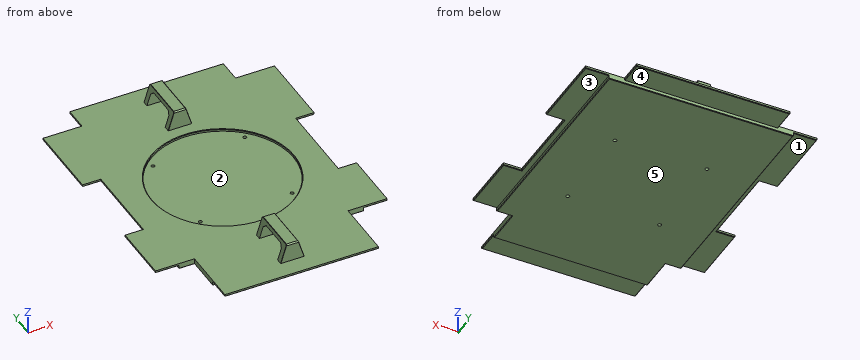
```python
from build123d import *
from OCP.BRepFilletAPI import BRepFilletAPI_MakeChamfer

# Parameters (mm, degrees)
SKETCH_1_W          = 156
SKETCH_1_H          = 185
EXTRUDE_1_DEPTH     = 3
SKETCH_2_W          = 130
SKETCH_2_H          = 30
EXTRUDE_2_DEPTH     = 3
EXTRUDE_3_DEPTH     = 2
SKETCH_4_W          = 15.5
SKETCH_4_H          = 50
SKETCH_4_H_2        = 65
EXTRUDE_4_DEPTH     = 2
SKETCH_5_R          = 1.5
CUT_EXTRUDE_1_DEPTH = 174.018062641
CHAMFER_1_SIZE      = 0.5
CHAMFER_2_SIZE      = 0.5
CHAMFER_3_SIZE      = 0.5
SKETCH_6_R          = 60
CUT_EXTRUDE_2_DEPTH = 2
CHAMFER_4_SIZE      = 0.5
EXTRUDE_5_DEPTH     = 10
CUT_EXTRUDE_3_DEPTH = 261.086524065
CHAMFER_5_SIZE      = 3
CHAMFER_6_SIZE      = 1
CHAMFER_7_SIZE      = 0.2
CHAMFER_7_SIZE2     = 0.159648139
CHAMFER_7_SIZE2_2   = 0.168291059
CHAMFER_7_SIZE2_3   = 0.304782811
CHAMFER_7_SIZE2_4   = 0.260894728


with BuildPart() as part:
    # 草图1 → 凸台-拉伸1 (new body)
    with BuildSketch(Plane.XY):
        Rectangle(SKETCH_1_W, SKETCH_1_H)
    extrude(amount=EXTRUDE_1_DEPTH)

    # 草图2 → 凸台-拉伸2 (add)
    with BuildSketch(Plane.XY.offset(3)):
        with Locations((0, -107.5)):
            Rectangle(SKETCH_2_W, SKETCH_2_H)
    extrude(amount=-EXTRUDE_2_DEPTH)

    # 草图3 → 凸台-拉伸3 (add)
    with BuildSketch(Plane.XY.offset(3)):
        Polygon((-82.5, 92.5), (-65, 92.5), (-65, 112.5), (65, 112.5), (65, 92.5), (82.5, 92.5), (82.5, -92.5), (65, -92.5), (65, -142.5), (-65, -142.5), (-65, -92.5), (-82.5, -92.5), align=None)
    extrude(amount=EXTRUDE_3_DEPTH)

    # 草图4 → 凸台-拉伸4 (add)
    with BuildSketch(Plane.XY.offset(5)):
        with Locations((-90.25, -67.5)):
            Rectangle(SKETCH_4_W, SKETCH_4_H)
        with Locations((-90.25, 60)):
            Rectangle(SKETCH_4_W, SKETCH_4_H_2)
        with Locations((90.25, 60)):
            Rectangle(SKETCH_4_W, SKETCH_4_H_2)
        with Locations((90.25, -67.5)):
            Rectangle(SKETCH_4_W, SKETCH_4_H)
    extrude(amount=-EXTRUDE_4_DEPTH)

    # 草图5 → 切除-拉伸1 (cut, through all)
    with BuildSketch(Plane.XY.offset(5)):
        with Locations((-38.890872965, 26.390872965)):
            Circle(SKETCH_5_R)
        with Locations((38.890872965, 26.390872965)):
            Circle(SKETCH_5_R)
        with Locations((38.890872965, -51.390872965)):
            Circle(SKETCH_5_R)
        with Locations((-38.890872965, -51.390872965)):
            Circle(SKETCH_5_R)
    extrude(amount=-CUT_EXTRUDE_1_DEPTH, mode=Mode.SUBTRACT)

    # 倒角1
    chamfer_1_edges = [part.edges().sort_by_distance(p)[0] for p in [
        (71.5, -92.5, 0),
        (-65, -107.5, 0),
        (65, -107.5, 0),
        (0, -122.5, 0),
        (0, 92.5, 0),
        (78, 0, 0),
        (-71.5, -92.5, 0),
        (-78, 0, 0),
    ]]
    chamfer(chamfer_1_edges, length=CHAMFER_1_SIZE)

    # 倒角2
    chamfer_2_edges = [part.edges().sort_by_distance(p)[0] for p in [
        (-88, 92.5, 3),
        (88, 92.5, 3),
        (-82.5, -7.5, 3),
        (-90.25, 27.5, 3),
        (-98, 60, 3),
        (-88, -92.5, 3),
        (-98, -67.5, 3),
        (-90.25, -42.5, 3),
        (98, 60, 3),
        (90.25, 27.5, 3),
        (82.5, -7.5, 3),
        (90.25, -42.5, 3),
        (98, -67.5, 3),
        (88, -92.5, 3),
        (-65, 102.5, 3),
        (65, 102.5, 3),
        (0, 112.5, 3),
        (0, -142.5, 3),
        (65, -132.5, 3),
    ]]
    chamfer(chamfer_2_edges, length=CHAMFER_2_SIZE)

    # 倒角3
    chamfer_3_edges = [part.edges().sort_by_distance(p)[0] for p in [
        (-65, -132.25, 3),
    ]]
    chamfer(chamfer_3_edges, length=CHAMFER_3_SIZE)

    # 草图6 → 切除-拉伸2 (cut)
    with BuildSketch(Plane.XY.offset(5)):
        with Locations((0, -12.5)):
            Circle(SKETCH_6_R)
    extrude(amount=-CUT_EXTRUDE_2_DEPTH, mode=Mode.SUBTRACT)

    # 倒角4
    chamfer_4_edges = [part.edges().sort_by_distance(p)[0] for p in [
        (-60, -12.5, 5),
    ]]
    chamfer(chamfer_4_edges, length=CHAMFER_4_SIZE)

    # 草图7 → 凸台-拉伸5 (add, symmetric)
    with BuildSketch(Plane(origin=(0, 0, 0), x_dir=(0, 0, -1), z_dir=(1, 0, 0))):
        Polygon((-5, 97.5), (-21, 97.5), (-21, 57.5), (-5, 57.5), (-5, 62.5), (-18, 62.5), (-18, 92.5), (-5, 92.5), align=None)
    extrude_5 = extrude(amount=EXTRUDE_5_DEPTH, both=True)

    # 草图8 → 切除-拉伸3 (cut, through all)
    with BuildSketch(Plane(origin=(0, 97.5, 0), x_dir=(1, 0, 0), z_dir=(0, 1, 0))):
        Polygon((-10, -5), (-5, -21), (-10, -21), align=None)
        Polygon((10, -5), (10, -21), (5, -21), align=None)
    cut_extrude_3 = extrude(amount=-CUT_EXTRUDE_3_DEPTH, mode=Mode.SUBTRACT)

    # 镜向2: 凸台-拉伸5, 切除-拉伸3 across plane
    add(extrude_5.mirror(Plane(origin=(0, -15, 0), x_dir=(0, 0, 1), z_dir=(0, -1, 0))))
    add(cut_extrude_3.mirror(Plane(origin=(0, -15, 0), x_dir=(0, 0, 1), z_dir=(0, -1, 0))), mode=Mode.SUBTRACT)

    # 倒角5
    chamfer_5_edges = [part.edges().sort_by_distance(p)[0] for p in [
        (0, 62.5, 18),
        (0, 92.5, 18),
        (0, -122.5, 18),
        (0, -92.5, 18),
    ]]
    chamfer(chamfer_5_edges, length=CHAMFER_5_SIZE)

    # 倒角6
    chamfer_6_edges = [part.edges().sort_by_distance(p)[0] for p in [
        (0, 97.5, 21),
        (0, 57.5, 21),
        (0, -87.5, 21),
        (0, -127.5, 21),
    ]]
    chamfer(chamfer_6_edges, length=CHAMFER_6_SIZE)

    # 倒角7: one chamfer whose edges measure the first distance from different faces: ONE call of the kernel's chamfer builder (chamfer() names one face for all edges)
    chamfer_7_edges_1 = [part.edges().sort_by_distance(p)[0] for p in [
        (-7.65625, 57.5, 12.5),
        (7.65625, 97.5, 12.5),
        (7.65625, -87.5, 12.5),
        (7.65625, -127.5, 12.5),
        (8.4375, -122.5, 10),
        (8.4375, -92.5, 10),
        (-7.65625, -87.5, 12.5),
        (-7.65625, -127.5, 12.5),
        (7.65625, 57.5, 12.5),
        (-7.65625, 97.5, 12.5),
    ]]
    chamfer_7_edges_2 = [part.edges().sort_by_distance(p)[0] for p in [
        (5.9375, -107.5, 18),
    ]]
    chamfer_7_side_2 = [part.faces().sort_by_distance(p)[0] for p in [
        (0, -107.5, 18),
    ]]
    chamfer_7_edges_3 = [part.edges().sort_by_distance(p)[0] for p in [
        (6.40625, -121, 16.5),
    ]]
    chamfer_7_side_3 = [part.faces().sort_by_distance(p)[0] for p in [
        (0, -121.036585366, 16.463414634),
    ]]
    chamfer_7_edges_4 = [part.edges().sort_by_distance(p)[0] for p in [
        (6.40625, -94, 16.5),
    ]]
    chamfer_7_side_4 = [part.faces().sort_by_distance(p)[0] for p in [
        (0, -93.963414634, 16.463414634),
    ]]
    chamfer_7_edges_5 = [part.edges().sort_by_distance(p)[0] for p in [
        (5, -107.5, 21),
    ]]
    chamfer_7_side_5 = [part.faces().sort_by_distance(p)[0] for p in [
        (0, -107.5, 21),
    ]]
    chamfer_7_edges_6 = [part.edges().sort_by_distance(p)[0] for p in [
        (5.15625, -127, 20.5),
        (-5.15625, -127, 20.5),
    ]]
    chamfer_7_side_6 = [part.faces().sort_by_distance(p)[0] for p in [
        (0, -127.005050505, 20.494949495),
    ]]
    chamfer_7_edges_7 = [part.edges().sort_by_distance(p)[0] for p in [
        (5.15625, -88, 20.5),
        (-5.15625, -88, 20.5),
    ]]
    chamfer_7_side_7 = [part.faces().sort_by_distance(p)[0] for p in [
        (0, -87.994949495, 20.494949495),
    ]]
    chamfer_7_edges_8 = [part.edges().sort_by_distance(p)[0] for p in [
        (-5, -107.5, 21),
    ]]
    chamfer_7_side_8 = [part.faces().sort_by_distance(p)[0] for p in [
        (-7.65625, -87.933704969, 12.5),
    ]]
    chamfer_7_edges_9 = [part.edges().sort_by_distance(p)[0] for p in [
        (-5, 77.5, 21),
    ]]
    chamfer_7_side_9 = [part.faces().sort_by_distance(p)[0] for p in [
        (0, 77.5, 21),
    ]]
    chamfer_7_edges_10 = [part.edges().sort_by_distance(p)[0] for p in [
        (5, 77.5, 21),
    ]]
    chamfer_7_side_10 = [part.faces().sort_by_distance(p)[0] for p in [
        (7.65625, 97.066295031, 12.5),
    ]]
    chamfer_7_edges_11 = [part.edges().sort_by_distance(p)[0] for p in [
        (5.15625, 97, 20.5),
        (-5.15625, 97, 20.5),
    ]]
    chamfer_7_side_11 = [part.faces().sort_by_distance(p)[0] for p in [
        (0, 97.005050505, 20.494949495),
    ]]
    chamfer_7_edges_12 = [part.edges().sort_by_distance(p)[0] for p in [
        (5.15625, 58, 20.5),
        (-5.15625, 58, 20.5),
    ]]
    chamfer_7_side_12 = [part.faces().sort_by_distance(p)[0] for p in [
        (0, 57.994949495, 20.494949495),
    ]]
    chamfer_7 = BRepFilletAPI_MakeChamfer(part.part.solid().wrapped)
    for e in chamfer_7_edges_1:
        chamfer_7.Add(CHAMFER_7_SIZE, e.wrapped)
    for e in chamfer_7_edges_2:
        chamfer_7.Add(CHAMFER_7_SIZE, CHAMFER_7_SIZE2, e.wrapped, chamfer_7_side_2[0].wrapped)  # the first distance lies on this face
    for e in chamfer_7_edges_3:
        chamfer_7.Add(CHAMFER_7_SIZE, CHAMFER_7_SIZE2_2, e.wrapped, chamfer_7_side_3[0].wrapped)  # the first distance lies on this face
    for e in chamfer_7_edges_4:
        chamfer_7.Add(CHAMFER_7_SIZE, CHAMFER_7_SIZE2_2, e.wrapped, chamfer_7_side_4[0].wrapped)  # the first distance lies on this face
    for e in chamfer_7_edges_5:
        chamfer_7.Add(CHAMFER_7_SIZE, CHAMFER_7_SIZE2_3, e.wrapped, chamfer_7_side_5[0].wrapped)  # the first distance lies on this face
    for e in chamfer_7_edges_6:
        chamfer_7.Add(CHAMFER_7_SIZE, CHAMFER_7_SIZE2_4, e.wrapped, chamfer_7_side_6[0].wrapped)  # the first distance lies on this face
    for e in chamfer_7_edges_7:
        chamfer_7.Add(CHAMFER_7_SIZE, CHAMFER_7_SIZE2_4, e.wrapped, chamfer_7_side_7[0].wrapped)  # the first distance lies on this face
    for e in chamfer_7_edges_8:
        chamfer_7.Add(CHAMFER_7_SIZE, CHAMFER_7_SIZE2_3, e.wrapped, chamfer_7_side_8[0].wrapped)  # the first distance lies on this face
    for e in chamfer_7_edges_9:
        chamfer_7.Add(CHAMFER_7_SIZE, CHAMFER_7_SIZE2_3, e.wrapped, chamfer_7_side_9[0].wrapped)  # the first distance lies on this face
    for e in chamfer_7_edges_10:
        chamfer_7.Add(CHAMFER_7_SIZE, CHAMFER_7_SIZE2_3, e.wrapped, chamfer_7_side_10[0].wrapped)  # the first distance lies on this face
    for e in chamfer_7_edges_11:
        chamfer_7.Add(CHAMFER_7_SIZE, CHAMFER_7_SIZE2_4, e.wrapped, chamfer_7_side_11[0].wrapped)  # the first distance lies on this face
    for e in chamfer_7_edges_12:
        chamfer_7.Add(CHAMFER_7_SIZE, CHAMFER_7_SIZE2_4, e.wrapped, chamfer_7_side_12[0].wrapped)  # the first distance lies on this face
    add(Compound.cast(chamfer_7.Shape()), mode=Mode.REPLACE)


solid = part.part
```
The model under review builds one solid part; all positions refer to its coordinate system, in mm. Face numbers are marked on the shaded views. A direction names the side the tool comes from. Coordinates: 2 decimals unless noted, no trailing zeros. Order: outer loops, then holes, each group sorted by start corner. A loop starts at its lowest first (then second) coordinate and runs counter-clockwise, first axis right, second up. Notation, with made-up numbers: (60, 24) -> (91, 24) arc R19 ccw to (91, 49) -> close; hole circle Ø7 at (11, 44). An arc over 180 degrees is marked (long way). Answer in a Markdown table with one row per item. Add a question column.
Item 1: We need section D-D on y = -12.5. Write out the cut boundary in (x, z), plus the area to 3 significant figures.
Item 2: To check wall thickness, follow probe 1 along Y at (x, z) = (-4, 6.75); probe 2 along Z at (x, y) = (2.5, 86); probe 3 along Z at (x, y) = (-57, -110). State the ranges of each line that lie inside material, in increasing order.
Item 3: Machinability: for the marked faces 3, 4 and 5, which of the approach directions +Z, -Z, +X, -X, +Y, -Y give a long, thin tool a straight path to every point of the face, cutting with its end or side? Answer none if there is none.
Item 4: We need section B-B on z = 12. Write out the cut boundary in (x, y), plus the area to 3 significant figures.
Item 5: We need section A-A on y = 72. Write out the cut boundary in (x, z), plus the area to 3 significant figures.
Item 6: Clearance check with flat-ended pins moving along their axes: pin 1 (1.3 mm diameter, centred on y = -113, z = 3.5, fed in from +X); pin 2 (5 mm diameter, centred on x = -1, z = 11.5, fed in from +Y); pin 3 (6 mm diameter, centred on x = 90.5, y = 43.5, fed in from -Z). State where each tip first meets the part, or that it passes through.
Item 7: Mouldability with a two-part tool opening along Y and no side actions: class the marked faces 1 and 2 as +Y half, -Y half, draft (parallel to the pull), parting line (faces both ways), or undercut.
Item 8: We need section C-C on x = 70. Write out the cut boundary in (y, z), plus the area to 3 significant figures.
Final values:
| question | item | result |
|---|---|---|
| 1 | outline | (-82.5, 3.5) -> (-82, 3) -> (-78, 3) -> (-78, 0.5) -> (-77.5, 0) -> (77.5, 0) -> (78, 0.5) -> (78, 3) -> (82, 3) -> (82.5, 3.5) -> (82.5, 5) -> (60.5, 5) -> (60, 4.5) -> (60, 3) -> (-60, 3) -> (-60, 4.5) -> (-60.5, 5) -> (-82.5, 5) -> close |
| 1 | area | 557 mm2 |
| 2 | probe 1 | y = -127.5 to -122.5, -92.5 to -87.5, 57.5 to 62.5, 92.5 to 97.5 |
| 2 | probe 2 | z = 0 to 5, 18 to 21 |
| 2 | probe 3 | z = 0 to 5 |
| 3 | face 3 | -Z, +X, +Y, -Y |
| 3 | face 4 | -Z, +X, -X, +Y |
| 3 | face 5 | -Z, +X, -X, +Y, -Y |
| 4 | outline | (-7.81, -127.3) -> (-7.6, -127.5) -> (7.6, -127.5) -> (7.81, -127.3) -> (7.81, -122.7) -> (7.6, -122.5) -> (-7.81, -122.5) -> close; (-7.81, -92.5) -> (7.6, -92.5) -> (7.81, -92.3) -> (7.81, -87.7) -> (7.6, -87.5) -> (-7.6, -87.5) -> (-7.81, -87.7) -> close; (-7.81, 57.7) -> (-7.6, 57.5) -> (7.6, 57.5) -> (7.81, 57.7) -> (7.81, 62.5) -> (-7.81, 62.5) -> close; (-7.81, 92.5) -> (7.81, 92.5) -> (7.81, 97.3) -> (7.6, 97.5) -> (-7.6, 97.5) -> (-7.81, 97.3) -> close |
| 4 | area | 312 mm2 |
| 5 | outline | (-98, 3.5) -> (-97.5, 3) -> (-78, 3) -> (-78, 0.5) -> (-77.5, 0) -> (77.5, 0) -> (78, 0.5) -> (78, 3) -> (97.5, 3) -> (98, 3.5) -> (98, 5) -> (-98, 5) -> close; (-5.94, 18) -> (5.94, 18) -> (5.06, 20.81) -> (4.7, 21) -> (-4.8, 21) -> (-5.09, 20.71) -> close |
| 5 | area | 892 mm2 |
| 6 | pin 1 | stops at x = 65 |
| 6 | pin 2 | stops at y = 97.5 |
| 6 | pin 3 | stops at z = 3 |
| 7 | face 1 | draft |
| 7 | face 2 | undercut |
| 8 | outline | (-92.5, 0.5) -> (-92, 0) -> (92, 0) -> (92.5, 0.5) -> (92.5, 5) -> (-92.5, 5) -> close |
| 8 | area | 925 mm2 |
